The listing builds one solid part. Answer for the finished solid, in the listing's coordinates (mm). Face numbers are marked on the shaded views. Coordinates: 2 decimals unless noted, no trailing zeros. Order: outer loops, then holes, each group sorted by start corner. A loop starts at its lowest first (then second) coordinate and runs counter-clockwise, first axis right, second up. Notation, with made-up numbers: (30.25, -38) - (80.25, -38) arc R27 cw to (80.25, -20) - close; hole circle Ø4 at (-39, 47). An arc over 180 degrees is marked (long way). One line per item, written item: value. Start each with the question number.
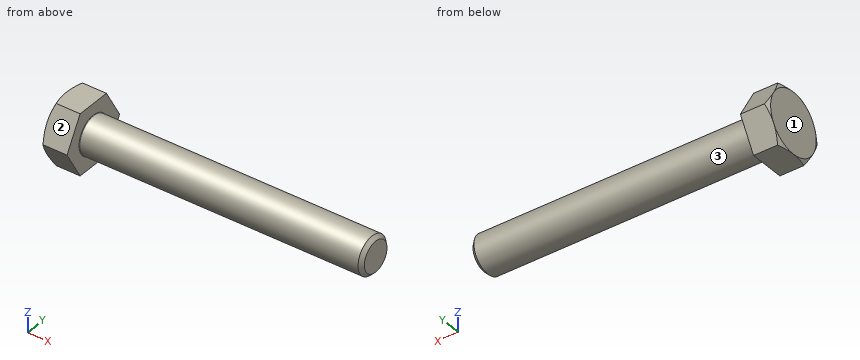
Autodesk Inventor part; units mm, degrees
ref_plane "Work Plane1" through (1.525, 0, 0) normal (0, 0, 1) x (1, 0, 0)
ref_plane "YZ Plane" through (0, 0, 0) normal (1, 0, 0) x (0, 1, 0)
ref_plane "XZ Plane" through (0, 0, 0) normal (0, 1, 0) x (-1, 0, 0)
sketch "Sketch1" plane through (0, 0, 0) normal (0, 0, 1) x (1, 0, 0)
  line L0 (0, 4) -> (60, 4)
  line L1 (60, 4) -> (60, 0)
  line L2 (60, 0) -> (0, 0)
  line L3 (-12, 0) -> (72, 0)
  line L4 (0, -0.8) -> (0, 4.8)
  line L5 (0, 4) -> (0, 0)
  dimension "d2" = 8
  dimension "d59" = 60
revolve "Body" add sketch "Sketch1" angle 360 about axis through (60, 0, 0) along (-1, 0, 0)
sketch "Sketch2" plane through (0, 0, 0) normal (-1, 0, 0) x (0, 0, 1)
  line L0 (0, 7.5056) -> (6.5, 3.7528)
  line L1 (6.5, 3.7528) -> (6.5, -3.7528)
  line L2 (6.5, -3.7528) -> (0, -7.5056)
  line L3 (0, -7.5056) -> (-6.5, -3.7528)
  line L4 (-6.5, -3.7528) -> (-6.5, 3.7528)
  line L5 (-6.5, 3.7528) -> (0, 7.5056)
  line L6 (-9.1, 0) -> (9.1, 0)
  line L7 (0, 10.5078) -> (0, -10.5078)
  point P0 (0, 0)
  point P1 (0, 0)
  dimension "d11" = 13
extrude "Head" add sketch "Sketch2" along normal blind 5.68
sketch "Sketch4" plane through (0, 0, 0) normal (0, 0, 1) x (1, 0, 0)
  line L0 (-4.9294, 7.8) -> (-5.68, 6.5)
  line L1 (-1.1, 0) -> (-0.234, 0)
  line L2 (-6.7692, 0) -> (0.8552, 0)
  line L3 (-5.68, 7.8) -> (-4.9294, 7.8)
  line L4 (-5.68, 6.5) -> (-5.68, 7.8)
  line L5 (0, 9.36) -> (0, -1.56)
  dimension "d65" = 13
  dimension "d67" = 30
  dimension "d68" = 15.6
  dimension "d69" = 5.68
revolve "Chamfer1" cut sketch "Sketch4" angle 360 about axis through (-1.1, 0, 0) along (1, 0, 0)
thread "Thread"
chamfer "Chamfer2" distance 0.7668 distance2 0.7669 1 edges at (60, -4, 0) measured on face at (60, -0.1514, -1.2467)
fillet "Fillet" radius 0.1 1 edges at (0, -4, 0)
ref_plane "Work Plane1" through (1.525, 0, 0) normal (0, 0, 1) x (1, 0, 0)
equation "\"d2\" = GD"
equation "\"d59\" = NLG"
equation "\"d11\" = SW"
equation "\"d3\" = KOH"
equation "\"d15\" = GEL"
equation "\"d6\" = -0.5 * SPD + 0.5 * GD"
equation "\"d71\" = RR"
equation "\"d65\" = SW"
equation "\"d67\" = ANG1"
equation "\"d68\" = 1.2 * SW"
equation "\"d69\" = KOH"
equation "\"NLG\" = 60"
equation "\"GD\" = NND"
equation "\"BDM\" = NND"
equation "\"KOH\" = 5.68"
equation "\"GEL\" = 22"
equation "\"SW\" = 13"
equation "\"SW0\" = SW"
equation "\"SPD\" = NND - 1.2269 * PTC"
equation "\"SD2\" = NND"
equation "\"SD\" = 0"
equation "\"ANG1\" = 30deg"
equation "\"GAL\" = 0.61345 * PTC"
equation "\"GUL\" = 0.61345 * PTC"
equation "\"RR\" = 0.1"
equation "\"RR1\" = 0.4"
equation "\"GD1\" = THREADDIA - 1.2269 * PTC"
equation "\"THREADDIA\" = 8"
equation "\"TOA\" = 30deg"
equation "\"PTC\" = 1.25"
equation "\"KOH1\" = 3.7"
equation "\"NND\" = 8"
equation "\"E0\" = 1.155 * SW"
properties part number "ANSI B18.2.3.5M - M8 x 1.25 x 60" material "Steel, Mild"
(1) For a pull along Y with two mould halves and no side action, classify the marked faces 1, 2 and 3 as pulls with the +Y half, pulls with the -Y half, needs draft (parallel to the pull), parting line crosses it, or undercut.
(2) Consider probe 1 along X at (y, z) = (1.25, 4.5); probe 2 along X at (y, z) = (2.5, 2.5); probe 3 along Y at (x, z) = (54.5, -0.75). Determine where each line is inside the solid, lowest interval first.
(3) The part is cut by section A-A on x = 29.5. Determine the outline of the cut face in (y, z).
(4) Flat-ended cylindrical pins translate along their axes: pin 1 Ø3 at (x, y) = (46, -0.5) entering from -Z; pin 2 Ø8 at (x, y) = (19, 0.5) entering from +Z; pin 3 Ø1 at (x, z) = (34, 1) entering from -Y; pin 4 Ø8 at (x, y) = (2, 6) entering from +Z. Find the tip coordinate at first contact, or state that the pin passes through.
Completed:
1. face 1: needs draft
1. face 2: pulls with the -Y half
1. face 3: parting line crosses it
2. probe 1: x = -5.68 to 0
2. probe 2: x = -5.68 to 59.7
2. probe 3: y = -3.93 to 3.93
3. outline: circle Ø8 at (0, 0)
4. pin 1: stops at z = -4
4. pin 2: stops at z = 4
4. pin 3: stops at y = -3.97
4. pin 4: stops at z = 6.5
